Part model, mm, in its own coordinate system. Face numbers are marked on the shaded views. A direction names the side the tool comes from. Give positions to 0.01 mm unless a question says otherwise; leave off trailing zeros. Order: outer loops, then holes, each group sorted by start corner. A loop starts at its lowest first (then second) coordinate and runs counter-clockwise, first axis right, second up. Notation, with made-up numbers: (75.25, 69) - (122.25, 69) arc R6 cw to (122.25, 76) - close; hole circle Ø5 at (-15, -15.5). An arc over 180 degrees is marked (long way). Use a Markdown table: item, result. Add a question column.
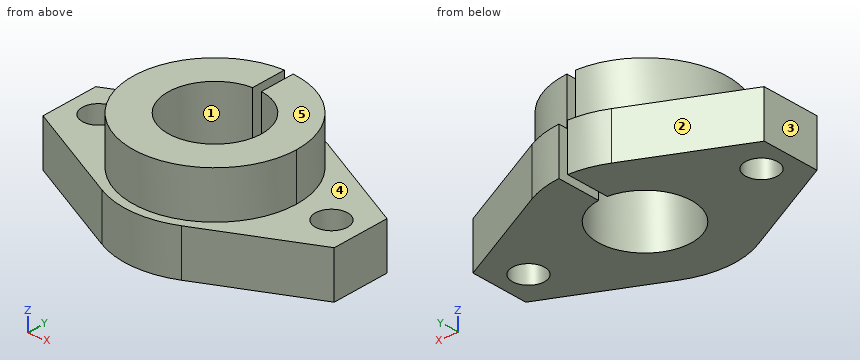
from build123d import *

# Parameters (mm, degrees)
BOSS_EXTRUDE1_DEPTH = 8
SKETCH2_R           = 14
BOSS_EXTRUDE2_DEPTH = 8
SKETCH3_R           = 8
CUT_EXTRUDE1_DEPTH  = 17
SKETCH4_R           = 2.75
CUT_EXTRUDE2_DEPTH  = 9
SKETCH5_W           = 1.5
SKETCH5_H           = 20
CUT_EXTRUDE3_DEPTH  = 17


with BuildPart() as part:
    # Sketch1 → Boss-Extrude1 (new body)
    with BuildSketch(Plane.XY):
        with BuildLine():
            Line((-6.826881704, 13.915591478), (-25, 5))
            Line((-25, 5), (-25, -5))
            Line((-25, -5), (-6.826881704, -13.915591478))
            ThreePointArc((-6.826881704, -13.915591478), (0, -15.5), (6.826881704, -13.915591478))
            Line((6.826881704, -13.915591478), (25, -5))
            Line((25, -5), (25, 5))
            Line((25, 5), (6.826881704, 13.915591478))
            ThreePointArc((6.826881704, 13.915591478), (0, 15.5), (-6.826881704, 13.915591478))
        make_face()
    extrude(amount=BOSS_EXTRUDE1_DEPTH)

    # Sketch2 → Boss-Extrude2 (add)
    with BuildSketch(Plane.XY.offset(8)):
        Circle(SKETCH2_R)
    extrude(amount=BOSS_EXTRUDE2_DEPTH)

    # Sketch3 → Cut-Extrude1 (cut, through all)
    with BuildSketch(Plane.XY.offset(16)):
        Circle(SKETCH3_R)
    extrude(amount=-CUT_EXTRUDE1_DEPTH, mode=Mode.SUBTRACT)

    # Sketch4 → Cut-Extrude2 (cut, through all)
    with BuildSketch(Plane.XY.offset(8)):
        with Locations((-20, 0)):
            Circle(SKETCH4_R)
        with Locations((20, 0)):
            Circle(SKETCH4_R)
    extrude(amount=-CUT_EXTRUDE2_DEPTH, mode=Mode.SUBTRACT)

    # Sketch5 → Cut-Extrude3 (cut, through all)
    with BuildSketch(Plane.XY.offset(16)):
        with Locations((0, 15)):
            Rectangle(SKETCH5_W, SKETCH5_H)
    extrude(amount=-CUT_EXTRUDE3_DEPTH, mode=Mode.SUBTRACT)


solid = part.part
1. Tool access for the marked faces 4 and 5: list every direction of +Z, -Z, +X, -X, +Y, -Y with a clear straight run to the whole face (end or side of a thin tool).
2. Cut at D-D (y = -11). Write the cut outline in (x, z).
3. Pin check, flat tips, straight feed: P1, Ø1, axis at x = 12, z = 7, coming from the -Y side; P2, Ø5, axis at x = 3.5, z = 13, coming from the -Y side; P3, Ø8, axis at x = -17.5, y = -6, coming from the +Z side. Stop position of each tip, or through.
4. Cut at C-C (x = 20). Write the cut outline in (y, z), plus the area to 3 significant figures.
5. Mould opens along Y. For the marked faces 1, 2 and 3 say: released by +Y, released by -Y, zero draft, split by the parting line, or undercut.
6. Cut at A-A (y = 12.5). Write the cut outline in (x, z).
7. Cut at B-B (z = 4.75). Write the cut outline in (x, y).
8. Drill centre lines: probe 1 along X at (y, z) = (0, 12.75); probe 2 along X at (y, z) = (5, 14.5) (3 decimals); probe 3 along Y at (x, z) = (2, 11). Where is each one in solid material? Low to high. Write a range as [from, to].
Responses:
| question | item | result |
|---|---|---|
| 1 | face 4 | +Z |
| 1 | face 5 | +Z, +X, -X, +Y, -Y |
| 2 | outline | (-12.77, 0) - (12.77, 0) - (12.77, 8) - (8.66, 8) - (8.66, 16) - (-8.66, 16) - (-8.66, 8) - (-12.77, 8) - close |
| 3 | P1 | stops at y = -11.62 |
| 3 | P2 | stops at y = -13.96 |
| 3 | P3 | stops at z = 8 |
| 4 | outline | (-7.45, 0) - (-2.75, 0) - (-2.75, 8) - (-7.45, 8) - close; (2.75, 0) - (7.45, 0) - (7.45, 8) - (2.75, 8) - close |
| 4 | area | 75.2 mm² |
| 5 | face 1 | undercut |
| 5 | face 2 | released by +Y |
| 5 | face 3 | zero draft |
| 6 | outline | (-9.71, 0) - (-0.75, 0) - (-0.75, 16) - (-6.3, 16) - (-6.3, 8) - (-9.71, 8) - close; (0.75, 0) - (9.71, 0) - (9.71, 8) - (6.3, 8) - (6.3, 16) - (0.75, 16) - close |
| 7 | outline | (-25, -5) - (-6.83, -13.92) arc R15.5 ccw to (6.83, -13.92) - (25, -5) - (25, 5) - (6.83, 13.92) arc R15.5 ccw to (0.75, 15.48) - (0.75, 7.96) arc R8 cw (long way) to (-0.75, 7.96) - (-0.75, 15.48) arc R15.5 ccw to (-6.83, 13.92) - (-25, 5) - close; hole circle Ø5.5 at (-20, 0); hole circle Ø5.5 at (20, 0) |
| 8 | probe 1 | x = [-14, -8], [8, 14] |
| 8 | probe 2 | x = [-13.077, -6.245], [6.245, 13.077] |
| 8 | probe 3 | y = [-13.86, -7.75], [7.75, 13.86] |
